Can you work these out from the model? Positions are in its coordinate system, mm. A direction names the side the tool comes from. Give positions to 0.01 mm unless a question says otherwise; leave off trailing zeros. Loops run counter-clockwise (first coordinate to the right, second up) from the corner with the lowest first, then second, coordinate; pieces in that order, holes last.
Autodesk Inventor part; units mm, degrees
ref_plane "YZ Plane" through (0, 0, 0) normal (1, 0, 0) x (0, 1, 0)
ref_plane "XZ Plane" through (0, 0, 0) normal (0, 1, 0) x (-1, 0, 0)
ref_plane "XY Plane" through (0, 0, 0) normal (0, 0, 1) x (1, 0, 0)
sketch "Sketch1" plane through (0, 0, 0) normal (0, 1, 0) x (-1, 0, 0)
  line L0 (28, 43) -> (-28, 43)
  line L1 (-28, 43) -> (-28, -43)
  line L2 (-28, -43) -> (28, -43)
  line L3 (28, -43) -> (28, 43)
  point P0 (0, 0)
  dimension "d0" = 56
  dimension "d1" = 86
  dimension "d4" = 28
  dimension "d5" = 43
extrude "Extrusion1" add sketch "Sketch1" along normal blind 7.5
sketch "Sketch3" plane through (0, 7.5, 0) normal (0, 1, 0) x (1, 0, 0)
  line L0 (22.5, -35) -> (27.5, -35)
  line L1 (27.5, -35) -> (27.5, -1.5)
  line L2 (27.5, -1.5) -> (22.5, -1.5)
  line L3 (22.5, -1.5) -> (22.5, -35)
  line L4 (-28, -43) -> (28, -43)
  line L5 (28, -43) -> (28, 43)
  point P0 (0, 0)
  dimension "d6" = 33.5
  dimension "d7" = 5
  dimension "d8" = 8
  dimension "d9" = 0.5
extrude "Extrusion2" add sketch "Sketch3" along normal blind 13.5
sketch "Sketch4" plane through (0, 7.5, 0) normal (0, 1, 0) x (1, 0, 0)
  line L0 (-28, 43) -> (-28, -43)
  line L1 (-30.4, -32.5) -> (-28, -32.5)
  line L2 (-28, -32.5) -> (-28, -22)
  line L3 (-28, -22) -> (-30.4, -22)
  line L4 (-30.4, -22) -> (-30.4, -32.5)
  line L5 (-30.4, 22.5) -> (-28, 22.5)
  line L6 (-28, 22.5) -> (-28, 33)
  line L7 (-28, 33) -> (-30.4, 33)
  line L8 (-30.4, 33) -> (-30.4, 22.5)
  line L9 (28, -43) -> (28, 43)
  line L10 (28, 22.5) -> (30.4, 22.5)
  line L11 (30.4, 22.5) -> (30.4, 33)
  line L12 (30.4, 33) -> (28, 33)
  line L13 (28, 33) -> (28, 22.5)
  line L14 (28, -32.5) -> (30.4, -32.5)
  line L15 (30.4, -32.5) -> (30.4, -22)
  line L16 (30.4, -22) -> (28, -22)
  line L17 (28, -22) -> (28, -32.5)
  line L18 (-28, -43) -> (28, -43)
  line L19 (28, 43) -> (-28, 43)
  point P0 (0, 0)
  dimension "d12" = 10.5
  dimension "d13" = 10.5
  dimension "d14" = 10.5
  dimension "d15" = 10
  dimension "d16" = 2.4
  dimension "d17" = 2.4
extrude "Extrusion3" add sketch "Sketch4" against normal blind 1.6 contours L0 L5 L8 L7 | L12 L11 L10 L9 | L0 L1 L4 L3 | L16 L15 L14 L9
sketch "Sketch5" plane through (0, 7.5, 0) normal (0, 1, 0) x (1, 0, 0)
  line L0 (-28, 43) -> (-28, -43)
  line L1 (28, -22) -> (28, 22.5)
  line L2 (-28, -43) -> (28, -43)
  line L3 (28, -43) -> (28, 18)
  line L4 (28, 18) -> (-28, 18)
  line L5 (-28, 18) -> (-28, -43)
  line L6 (28, 43) -> (-28, 43)
  point P0 (0, 0)
  dimension "d20" = 25
extrude "Extrusion4" add sketch "Sketch5" along normal blind 6.5
properties part number "Screen_Model"
(1) Suppose I cut it at D-D on z = 19. List the corners of the cut face in (x, y) for me.
Returned:
outline: (-28, 0) - (28, 0) - (28, 14) - (27.5, 14) - (27.5, 21) - (22.5, 21) - (22.5, 14) - (-28, 14) - close
(2) Suppose I cut it at B-B on y = 18.5. List the corners of the cut face in (x, z) for me.
Returned:
outline: (22.5, 1.5) - (27.5, 1.5) - (27.5, 35) - (22.5, 35) - close
(3) Will these pins go through, and if not, where does the flat tip stop? P1, Ø5, axis at x = 13.5, y = 13, coming from the -Z side; P2, Ø5.5, axis at x = 25, y = 18, coming from the -Z side; P3, Ø1.8, axis at x = 29, y = 6.5, coming from the -Z side.
Returned:
P1: stops at z = -18
P2: stops at z = 1.5
P3: stops at z = -33
(4) Please list where these lines run through material, in increasing order: probe 1 along X at (y, z) = (7, 21.5); probe 2 along Z at (x, y) = (10, 12); probe 3 along Y at (x, z) = (-1, 7).
Returned:
probe 1: x = -28 to 28
probe 2: z = -18 to 43
probe 3: y = 0 to 14
(5) Suppose I cut it at A-A on z = -24. List the corners of the cut face in (x, y) for me, plus the area to 3 significant figures.
Returned:
outline: (-30.4, 5.9) - (-28, 5.9) - (-28, 0) - (28, 0) - (28, 5.9) - (30.4, 5.9) - (30.4, 7.5) - (-30.4, 7.5) - close
area: 428 mm2
(6) Which directions (+Z, -Z, +X, -X, +Y, -Y) give clear straight access to the entire face, cutting with the end or side of a thin tool? Please do faces 1 (the flat face through (29, 5.9, -28)), 2 (the flat face through (-29, 7.5, 27)), 3 (the flat face through (-29, 5.9, -28)), 4 (the flat face through (25, 17, 1.5)), 5 (the flat face through (27.5, 17, 18)).
Returned:
face 1: +Z, -Z, +X, -Y
face 2: +Z, -Z, -X, +Y
face 3: +Z, -Z, -X, -Y
face 4: -Z, +X, -X, +Y
face 5: +Z, -Z, +X, +Y
(7) Suppose I cut it at C-C on x = 15.5. List the corners of the cut face in (y, z) for me.
Returned:
outline: (0, -43) - (7.5, -43) - (7.5, -18) - (14, -18) - (14, 43) - (0, 43) - close
